The figure shows three views and two pictorial views of one solid part (mm, origin at its lowest corner). Answer the questions. Round coordinates to 2 decimals unless told otherwise and drop trailing zeros. Order: outer loops, then holes, each group sorted by start corner. A loop starts at its lowest first (then second) coordinate and runs counter-clockwise, first axis right, second up. Notation, with made-up numbers: (87, 8.25) - (96, 8.25) arc R14 cw to (96, 32.25) - close; hole circle Ø8 at (56.5, 9.5). An arc over 180 degrees is marked (long way). Answer in a Markdown table with one row per item.
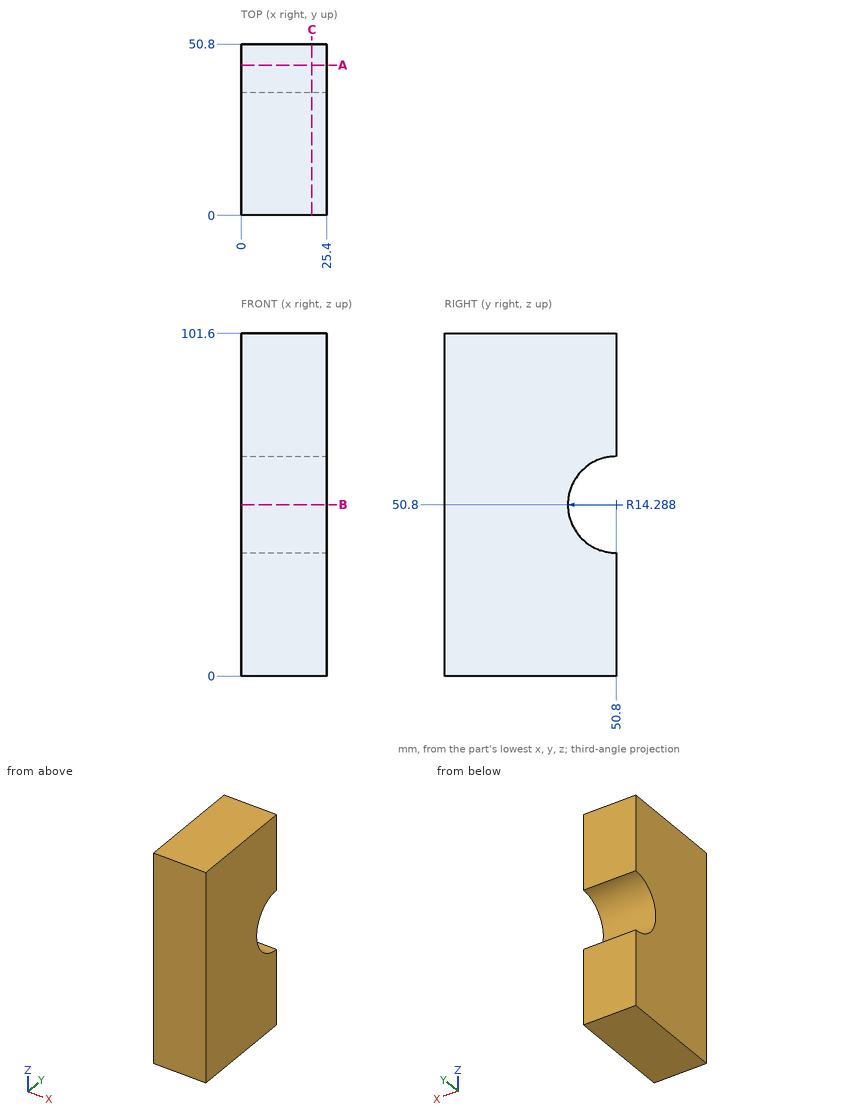
1) Find section C-C, the plane x = 21. Give the vertices of the cut face in (y, z) (1 decimal), then the cut area to 3 significant figures.
Filled in:
| item | result |
|---|---|
| outline | (0, 0) - (50.8, 0) - (50.8, 36.5) arc R14.3 cw to (50.8, 65.1) - (50.8, 101.6) - (0, 101.6) - close |
| area | 4,840 mm^2 |
2) Find section A-A, the plane y = 44.5. Give the vertices of the cut face in (x, z).
Filled in:
| item | result |
|---|---|
| outline | (0, 0) - (25.4, 0) - (25.4, 37.98) - (0, 37.98) - close; (0, 63.62) - (25.4, 63.62) - (25.4, 101.6) - (0, 101.6) - close |
3) Find the intervals of material crossed by probe 1 along Y at (x, z) = (23.75, 51.5); probe 2 along Z at (x, y) = (10.25, 42) (1 decimal); probe 3 along Y at (x, z) = (6.75, 62.5), in increasing order. Write a range as from..to.
Filled in:
| item | result |
|---|---|
| probe 1 | y = 0..36.53 |
| probe 2 | z = 0..39.5, 62.1..101.6 |
| probe 3 | y = 0..42.6 |
4) Find section B-B, the plane z = 50.8. Give the vertices of the cut face in (x, y).
Filled in:
| item | result |
|---|---|
| outline | (0, 0) - (25.4, 0) - (25.4, 36.51) - (0, 36.51) - close |
